Can you work these out from the model? Positions are in its coordinate system, mm. A direction names the side the tool comes from. Give positions to 0.01 mm unless a question says otherwise; leave off trailing zeros. Order: outer loops, then holes, each group sorted by start corner. A loop starts at its lowest first (then second) coordinate and runs counter-clockwise, first axis right, second up. Notation, with made-up numbers: M -14.75,-14.5 L 14.25,-14.5 A9 ccw 14.25,2.5 Z; hole C -9,69 d1. An arc over 180 degrees is marked long. Use a Markdown table: item, result. Add a question column.
from build123d import *

# Parameters (mm, degrees)
EXTRUDE_1_DEPTH = 2


with BuildPart() as part:
    # 草图1 → 凸台-拉伸1 (new body)
    with BuildSketch(Plane(origin=(0, 0, 0), x_dir=(1, 0, 0), z_dir=(0, 1, 0))):
        with BuildLine():
            Line((-26, 99.664436987), (-26, 96.560861637))
            Line((-26, 96.560861637), (-26, 92.533119315))
            ThreePointArc((-26, 92.533119315), (-35.261557972, 85.02385236), (-42.435244785, 75.5))
            Line((-42.435244785, 75.5), (-22.516660498, 64))
            ThreePointArc((-22.516660498, 64), (0, 77), (22.516660498, 64))
            Line((22.516660498, 64), (42.435244785, 75.5))
            ThreePointArc((42.435244785, 75.5), (35.261557972, 85.02385236), (26, 92.533119315))
            Line((26, 92.533119315), (26, 96.560861637))
            Line((26, 96.560861637), (26, 99.664436987))
            ThreePointArc((26, 99.664436987), (0, 103), (-26, 99.664436987))
        make_face()
    extrude(amount=EXTRUDE_1_DEPTH)


solid = part.part
1. If we section it at C-C, the plane z = -94.5: List the corners of the cut face in (x, y) for me, then the cut area to 3 significant figures.
2. Will these pins go through, and if not, where does the flat tip stop? pin 1 (1 mm diameter, centred on y = 1.5, z = -94.5, fed in from -X); pin 2 (1.5 mm diameter, centred on x = -21, z = -70.5, fed in from -Y).
3. If we section it at B-B, the plane y = 0.5: List the corners of the cut face in (x, z) for me.
4. If we section it at D-D, the plane x = -2.5: List the corners of the cut face in (y, z) for me.
5. I need wall thicknesses on L1, parallel to X at y = 1.35, z = -74; L2, parallel to Z at x = -29.5, y = 0.65; L3, parallel to Z at x = 4.5, y = 0.85. Which ranges of each line are inside material? Lowest first, please. Write a range as [from, to].
6. On a 3-axis mill with a long thin cutter (end or side, diameter ignored), from which of +Z, -Z, +X, -X, +Y, -Y can I reach the whole of each face in a straight line? I mean faces 1 (the face through (-32.615, 0.986, -69.83)), 2 (the face through (26, 1, -96)), 3 (the face through (-26, 1, -96)). Say none if no direction works.
7. If we section it at A-A, the plane z = -68: List the corners of the cut face in (x, y) for me, then the cut area to 3 significant figures.
Geometry results:
| question | item | result |
|---|---|---|
| 1 | outline | M -26,0 L 26,0 L 26,2 L -26,2 Z |
| 1 | area | 104 mm^2 |
| 2 | pin 1 | stops at x = -26 |
| 2 | pin 2 | stops at y = 0 |
| 3 | outline | M -42.44,-75.5 A49 ccw -26,-92.53 L -26,-99.66 A103 ccw 26,-99.66 L 26,-92.53 A49 ccw 42.44,-75.5 L 22.52,-64 A26 cw -22.52,-64 Z |
| 4 | outline | M 0,-102.97 L 2,-102.97 L 2,-76.88 L 0,-76.88 Z |
| 5 | L1 | x = [-39.84, -12.12], [12.12, 39.84] |
| 5 | L2 | z = [-90.12, -68.03] |
| 5 | L3 | z = [-102.9, -76.61] |
| 6 | face 1 | +Z, -X, +Y, -Y |
| 6 | face 2 | -Z, +X, +Y, -Y |
| 6 | face 3 | -Z, -X, +Y, -Y |
| 7 | outline | M -29.44,0 L -19.67,0 L -19.67,2 L -29.44,2 Z; M 19.67,0 L 29.44,0 L 29.44,2 L 19.67,2 Z |
| 7 | area | 39.1 mm^2 |
